from build123d import *

# Parameters (mm, degrees)
F0_W     = 100
F0_H     = 100
F1_DEPTH = 50
F2_SIZE  = 10
F4_D     = 5
F4_DEPTH = 12
F4_TIP   = 1.5021515476


with BuildPart() as f1:
    # F0 (on Front) → F1 (new body, symmetric)
    with BuildSketch(Plane.XZ):
        Rectangle(F0_W, F0_H)
    extrude(amount=F1_DEPTH, both=True)

    # F2
    f2_edges = [f1.edges().sort_by_distance(p)[0] for p in [
        (-50, 0, 50),
        (0, -50, 50),
        (50, 0, 50),
        (0, 50, 50),
        (50, -50, 0),
        (50, 50, 0),
        (-50, 50, 0),
        (-50, -50, 0),
    ]]
    chamfer(f2_edges, length=F2_SIZE)

    # F4
    with Locations(Plane(origin=(0, 0, -50), x_dir=(1, 0, 0), z_dir=(0, 0, -1))):
        with Locations((0, -35)):
            Hole(F4_D / 2, depth=F4_DEPTH)
            with Locations((0, 0, -(F4_DEPTH + F4_TIP / 2))):  # 118° drill point
                Cone(0, F4_D / 2, F4_TIP, mode=Mode.SUBTRACT)


solid = f1.part
Work out the finished part from the listing and answer in its coordinate system (mm). Give positions to 0.01 mm unless a question says otherwise; leave off trailing zeros. Order: outer loops, then holes, each group sorted by start corner. A loop starts at its lowest first (then second) coordinate and runs counter-clockwise, first axis right, second up. Notation, with made-up numbers: (84.25, 55.25) - (135.25, 55.25) arc R31 cw to (135.25, 79.25) - close; hole circle Ø10 at (-29.5, 79). An arc over 180 degrees is marked (long way). Answer as CSV lines item,"result". Start each with the question number.
Q1. The part is cut by section B-B (x = 44.5). Write down the section's boundary in (y, z).
Q2. The part is cut by section C-C (z = 42). Write down the section's boundary in (x, y).
Q3. The mould has two halves that part along X. Classify faces 1 (the face through (-1.34, 32.89, -43.92)), 2 (the face through (44, -43, 43)), 3 (the face through (-0.06, 34.57, -36.76)), 4 (the face through (-45, 45, -6)): +X half, -X half, draft (parallel to the pull), parting line (faces both ways), or undercut.
Q4. Given pin 1 Ø3 at (x, y) = (0, 35) entering from -Z, flat-ended and moving along its own axis, determine where the tip first touches the part or whether it passes through.
Q5. Find the intervals of material crossed by L1, parallel to X at y = 35, z = -42.5; L2, parallel to Y at x = 0, z = -43.5; L3, parallel to X at y = 34.5, z = -42.5, in increasing order. Write a range as [from, to].
Q6. The part is cut by section A-A (z = -31). Write down the section's boundary in (x, y), then the cut area to 3 significant figures.
Check result:
1,outline,"(-45.5, -50) - (45.5, -50) - (45.5, 40) - (40, 45.5) - (-40, 45.5) - (-45.5, 40) - close"
2,outline,"(-48, -40) - (-40, -48) - (40, -48) - (48, -40) - (48, 40) - (40, 48) - (-40, 48) - (-48, 40) - close"
3,face 1,"undercut"
3,face 2,"+X half"
3,face 3,"undercut"
3,face 4,"-X half"
4,pin 1,"stops at z = -37.4"
5,L1,"x = [-50, -2.5], [2.5, 50]"
5,L2,"y = [-50, 32.5], [37.5, 50]"
5,L3,"x = [-50, -2.45], [2.45, 50]"
6,outline,"(-50, -40) - (-40, -50) - (40, -50) - (50, -40) - (50, 40) - (40, 50) - (-40, 50) - (-50, 40) - close"
6,area,"9,800 mm²"
